Autodesk Fusion 360 part; units mm, degrees
sketch "Sketch1" plane through (0, 0, 0) normal (0, 1, 0) x (1, 0, 0)
  line L0 (-300, 30.15) -> (274, 30.15)
  line L1 (274, 30.15) -> (274, -30.15)
  line L2 (274, -30.15) -> (-300, -30.15)
  line L3 (-300, -30.15) -> (-300, 30.15)
  dimension "d1" = 574
  dimension "d2" = 60.3
  dimension "d3" = 300
  dimension "d4" = 30.15
extrude "Extrude1" add sketch "Sketch1" along normal blind 12
sketch "Sketch2" plane through (0, 12, 0) normal (0, 1, 0) x (-1, 0, 0)
  circle A0 centre (256.6, 26.25) radius 2
  line L0 (300, 30.15) -> (-274, 30.15)
  line L1 (300, -30.15) -> (300, 30.15)
  line L2 (256.6, 26.25) -> (294.4, 26.25) construction
  line L3 (294.4, 26.25) -> (294.4, -26.25) construction
  line L4 (294.4, -26.25) -> (256.6, -26.25) construction
  line L5 (256.6, -26.25) -> (256.6, 26.25) construction
  circle A1 centre (294.4, -26.25) radius 2
  circle A2 centre (256.6, -26.25) radius 2
  circle A3 centre (294.4, 26.25) radius 2
  dimension "d9" = 4
  dimension "d13" = 52.5
  dimension "d14" = 37.8
  dimension "d15" = 26.25
  dimension "d16" = 5.6
  dimension "d17" = 4
  dimension "d18" = 4
  dimension "d19" = 4
extrude "Extrude2" cut sketch "Sketch2" against normal through all
sketch "Sketch3" plane through (0, 12, 0) normal (0, 1, 0) x (-1, 0, 0)
  circle A0 centre (256.6, 26.25) radius 2
  line L0 (300, 30.15) -> (-274, 30.15)
  line L1 (-274, 30.15) -> (-274, -30.15)
  line L2 (-274, -30.15) -> (300, -30.15)
  line L3 (300, -30.15) -> (300, 30.15)
  circle A1 centre (256.6, -26.25) radius 2
  circle A2 centre (294.4, -26.25) radius 2
  circle A3 centre (294.4, 26.25) radius 2
sketch "Sketch4" plane through (0, 12, 0) normal (0, 1, 0) x (-1, 0, 0)
  line L0 (300, 30.15) -> (-274, 30.15)
  line L1 (-274, 30.15) -> (-274, -30.15)
  line L2 (-274, -30.15) -> (300, -30.15)
  line L3 (300, -30.15) -> (300, 30.15)
  circle A0 centre (256.6, -26.25) radius 2
  circle A1 centre (294.4, -26.25) radius 2
  circle A2 centre (256.6, 26.25) radius 2
  circle A3 centre (294.4, 26.25) radius 2
  circle A4 centre (-270, -26.25) radius 2
  circle A5 centre (-270, 26.25) radius 2
  dimension "d21" = 4
  dimension "d22" = 4
  dimension "d23" = 52.5
  dimension "d26" = 4
  dimension "d27" = 4
  dimension "d30" = 26.25
extrude "Extrude4" cut sketch "Sketch4" against normal through all contours A4 | A5
sketch "Sketch5" plane through (0, 12, 0) normal (0, 1, 0) x (-1, 0, 0)
  circle A0 centre (-270, -26.25) radius 2
  circle A1 centre (-270, 26.25) radius 2
  line L0 (-274, -30.15) -> (300, -30.15)
  line L1 (300, -30.15) -> (300, 30.15)
  line L2 (300, 30.15) -> (-274, 30.15)
  line L3 (-274, 30.15) -> (-274, -30.15)
  circle A2 centre (256.6, -26.25) radius 2
  circle A3 centre (294.4, -26.25) radius 2
  circle A4 centre (256.6, 26.25) radius 2
  circle A5 centre (294.4, 26.25) radius 2
  line L4 (240, 0) -> (-260, 0) construction
  circle A6 centre (230, 0) radius 1.5
  circle A7 centre (205, 0) radius 1.5
  circle A8 centre (180, 0) radius 1.5
  circle A9 centre (155, 0) radius 1.5
  circle A10 centre (130, 0) radius 1.5
  circle A11 centre (105, 0) radius 1.5
  circle A12 centre (80, 0) radius 1.5
  circle A13 centre (55, 0) radius 1.5
  circle A14 centre (30, 0) radius 1.5
  circle A15 centre (5, 0) radius 1.5
  circle A16 centre (-20, 0) radius 1.5
  circle A17 centre (-45, 0) radius 1.5
  circle A18 centre (-70, 0) radius 1.5
  circle A19 centre (-95, 0) radius 1.5
  circle A20 centre (-120, 0) radius 1.5
  circle A21 centre (-145, 0) radius 1.5
  circle A22 centre (-170, 0) radius 1.5
  circle A23 centre (-195, 0) radius 1.5
  circle A24 centre (-220, 0) radius 1.5
  circle A25 centre (-245, 0) radius 1.5
  dimension "d34" = 60
  dimension "d35" = 10
  dimension "d36" = 3
  dimension "d39" = -25
  dimension "d40" = 0
  dimension "d41" = 500
  dimension "d42" = 25
  dimension "d43" = 15
extrude "Extrude5" cut sketch "Sketch5" against normal through all contours A6 | A7 | A8 | A9 | A10 | A11 | A12 | A13 | A14 | A15 | A16 | A17 | A18 | A19 | A20 | A21 | A22 | A23 | A24 | A25
sketch "Sketch6" plane through (0, 0, 0) normal (0, -1, 0) x (1, 0, 0)
  circle A0 centre (195, 0) radius 1.5
  circle A1 centre (95, 0) radius 1.5
  circle A2 centre (-5, 0) radius 1.5
  circle A3 centre (-105, 0) radius 1.5
  circle A4 centre (-205, 0) radius 1.5
  circle A5 centre (-180, 0) radius 1.5
  circle A6 centre (-80, 0) radius 1.5
  circle A7 centre (20, 0) radius 1.5
  circle A8 centre (120, 0) radius 1.5
  circle A9 centre (220, 0) radius 1.5
  circle A10 centre (170, 0) radius 1.5
  circle A11 centre (70, 0) radius 1.5
  circle A12 centre (-30, 0) radius 1.5
  circle A13 centre (-130, 0) radius 1.5
  circle A14 centre (-230, 0) radius 1.5
  circle A15 centre (-155, 0) radius 1.5
  circle A16 centre (-55, 0) radius 1.5
  circle A17 centre (45, 0) radius 1.5
  circle A18 centre (145, 0) radius 1.5
  circle A19 centre (245, 0) radius 1.5
  circle A20 centre (270, -26.25) radius 2
  circle A21 centre (270, 26.25) radius 2
  circle A22 centre (-256.6, -26.25) radius 2
  circle A23 centre (-294.4, -26.25) radius 2
  circle A24 centre (-256.6, 26.25) radius 2
  circle A25 centre (-294.4, 26.25) radius 2
  line L0 (274, -30.15) -> (274, 30.15)
  line L1 (274, 30.15) -> (-300, 30.15)
  line L2 (-300, 30.15) -> (-300, -30.15)
  line L3 (-300, -30.15) -> (274, -30.15)
  line L4 (-292, 10) -> (-263, 10)
  line L5 (-260, 7) -> (-260, -7)
  line L6 (-263, -10) -> (-292, -10)
  line L7 (-295, -7) -> (-295, 7)
  arc A26 (-292, 10) -> (-295, 7) centre (-292, 7) ccw
  arc A27 (-260, 7) -> (-263, 10) centre (-263, 7) ccw
  arc A28 (-263, -10) -> (-260, -7) centre (-263, -7) ccw
  arc A29 (-295, -7) -> (-292, -10) centre (-292, -7) ccw
  dimension "d45" = 20.15
  dimension "d46" = 20
  dimension "d47" = 35
  dimension "d48" = 5
  dimension "d49" = 3
  dimension "d50" = 3
extrude "Extrude6" cut sketch "Sketch6" against normal through all contours L4 L5 L6 L7 A26 A27 A28 A29
sketch "Sketch8" plane through (0, 0, 0) normal (0, -1, 0) x (1, 0, 0)
  line L0 (-260, 7) -> (-260, -7)
  arc A0 (-263, -10) -> (-260, -7) centre (-263, -7) ccw
  line L1 (-263, -10) -> (-292, -10)
  arc A1 (-295, -7) -> (-292, -10) centre (-292, -7) ccw
  line L2 (-295, -7) -> (-295, 7)
  arc A2 (-292, 10) -> (-295, 7) centre (-292, 7) ccw
  line L3 (-292, 10) -> (-263, 10)
  arc A3 (-260, 7) -> (-263, 10) centre (-263, 7) ccw
  circle A4 centre (195, 0) radius 1.5
  circle A5 centre (95, 0) radius 1.5
  circle A6 centre (-5, 0) radius 1.5
  circle A7 centre (-105, 0) radius 1.5
  circle A8 centre (-205, 0) radius 1.5
  circle A9 centre (-180, 0) radius 1.5
  circle A10 centre (-80, 0) radius 1.5
  circle A11 centre (20, 0) radius 1.5
  circle A12 centre (120, 0) radius 1.5
  circle A13 centre (220, 0) radius 1.5
  circle A14 centre (170, 0) radius 1.5
  circle A15 centre (70, 0) radius 1.5
  circle A16 centre (-30, 0) radius 1.5
  circle A17 centre (-130, 0) radius 1.5
  circle A18 centre (-230, 0) radius 1.5
  circle A19 centre (-155, 0) radius 1.5
  circle A20 centre (-55, 0) radius 1.5
  circle A21 centre (45, 0) radius 1.5
  circle A22 centre (145, 0) radius 1.5
  circle A23 centre (245, 0) radius 1.5
  circle A24 centre (270, -26.25) radius 2
  circle A25 centre (270, 26.25) radius 2
  circle A26 centre (-256.6, -26.25) radius 2
  circle A27 centre (-294.4, -26.25) radius 2
  circle A28 centre (-256.6, 26.25) radius 2
  circle A29 centre (-294.4, 26.25) radius 2
  line L4 (274, -30.15) -> (274, 30.15)
  line L5 (274, 30.15) -> (-300, 30.15)
  line L6 (-300, 30.15) -> (-300, -30.15)
  line L7 (-300, -30.15) -> (274, -30.15)
  circle A30 centre (-230, 0) radius 1.5
  line L8 (-237.5, 3.05) -> (252.5, 3.05)
  line L9 (252.5, 3.05) -> (252.5, -3.05)
  line L10 (252.5, -3.05) -> (-237.5, -3.05)
  line L11 (-237.5, -3.05) -> (-237.5, 3.05)
  line L12 (242.25, 2.75) -> (247.75, 2.75) construction
  line L13 (247.75, 2.75) -> (247.75, -2.75) construction
  line L14 (247.75, -2.75) -> (242.25, -2.75) construction
  line L15 (242.25, -2.75) -> (242.25, 2.75) construction
  circle A31 centre (249.5, 0.05) radius 3 construction
  line L16 (-232.75, 2.75) -> (-227.25, 2.75) construction
  line L17 (-227.25, 2.75) -> (-227.25, -2.75) construction
  line L18 (-227.25, -2.75) -> (-232.75, -2.75) construction
  line L19 (-232.75, -2.75) -> (-232.75, 2.75) construction
  dimension "d54" = 490
  dimension "d55" = 6.1
  dimension "d56" = 3.05
  dimension "d57" = 7.5
  dimension "d64" = 5.5
  dimension "d65" = 5.5
  dimension "d66" = 2.75
  dimension "d67" = 2.75
  dimension "d68" = 6
  dimension "d69" = 90
  dimension "d70" = 90
  dimension "d71" = 90
  dimension "d72" = 90
  dimension "d73" = 5.5
  dimension "d74" = 2.75
  dimension "d75" = 5.5
  dimension "d76" = 2.75
extrude "Extrude7" cut sketch "Sketch8" against normal blind 3 contours L8 L9 L10 L11
extrude "Extrude8" cut 1 faces at (-235.5, 3, 0) along direction (0, 1, 0) blind 3
hole "Hole3" at (242.5, 0, 7) direction (0, 1, 0) diameter 3 depth 10 tip angle 180
hole "Hole4" at (-227.5, 0, 7) direction (0, 1, 0) diameter 3 depth 10 tip angle 180
hole "Hole5" at (242.5, 0, -7) direction (0, 1, 0) diameter 3 depth 10 tip angle 180
hole "Hole6" at (-227.5, 0, -7) direction (0, 1, 0) diameter 3 depth 10 tip angle 180
equation "d1 = 600 mm - 19 mm - 7 mm"
equation "d4 = ( 60.3 / 2 ) * 1 mm"
equation "d15 = ( 52.5 / 2 ) * 1 mm"
equation "d34 = 75 mm - 15 mm"
equation "d56 = ( 6.1 / 2 ) * 1 mm"
equation "d66 = ( 5.5 / 2 ) * 1 mm"
equation "d67 = ( 5.5 / 2 ) * 1 mm"
equation "d74 = ( 5.5 / 2 ) * 1 mm"
equation "d76 = ( 5.5 / 2 ) * 1 mm"
equation "dbToolDia = 3 mm"
equation "dbOffset = 0 mm"
equation "dbRadius = ( dbToolDia + dbOffset ) / 2"
equation "dbHoleOffset = dbRadius / sqrt(2)"
equation "d91 = dbRadius * 2"
equation "d93 = dbHoleOffset"
equation "d94 = dbHoleOffset"
equation "d96 = dbRadius * 2"
equation "d98 = dbHoleOffset"
equation "d99 = dbHoleOffset"
equation "d101 = dbRadius * 2"
equation "d103 = dbHoleOffset"
equation "d104 = dbHoleOffset"
equation "d106 = dbRadius * 2"
equation "d108 = dbHoleOffset"
equation "d109 = dbHoleOffset"
Design review of the part built by this model. Coordinates are the model's own, in mm. A direction names the side the tool comes from. Coordinates: 2 decimals unless noted, no trailing zeros. Order: outer loops, then holes, each group sorted by start corner. A loop starts at its lowest first (then second) coordinate and runs counter-clockwise, first axis right, second up. Notation, with made-up numbers: (89.25, -8) -> (136.25, -8) arc R30 ccw to (136.25, 20) -> close; hole circle Ø6 at (76.5, 40.25). An arc over 180 degrees is marked (long way). One line per item, written item: value. Start each with the question number.
Q1. Take a section at B-B, the plane x = 204.5. State the section outline as (y, z) points, then the cut area to 3 significant figures.
Q2. Mouldability with a two-part tool opening along X and no side actions: class faces 3 (the flat face through (-9, 6, 30.15)), 4 (the flat face through (-300, 6, 0)), 5 (the flat face through (-278, 6, 10)) as pulls with the +X half, pulls with the -X half, needs draft (parallel to the pull), parting line crosses it, or undercut.
Q3. Insertion check: pin 1 Ø1.5 at (x, z) = (2, 1.5) entering from -Y; pin 2 Ø2.5 at (x, z) = (145, 0) entering from +Y. Each pin has a flat end and moves straight along its axis. Give the tip position at first contact, or say it passes through.
Q4. Tool access review of faces 1 (the flat face through (-17, 0, -7)), 2 (the flat face through (-295, 6, 0)): name each direction out of +Z, -Z, +X, -X, +Y, -Y from which nothing blocks a thin tool from reaching the whole face with its end or side.
Q5. Take a section at A-A, the plane y = 3.5. Give the number of separate pieces and of enclosed holes in the cut face, then the cut area to 3 significant figures.
Q6. For probe 1 along Z at (x, y) = (242.5, 5); probe 2 along X at (y, z) = (7.5, 7); probe 3 along X at (y, z) = (2.75, 3), list the stretches that pass through material, from the lowest coordinate up.
Values follow:
1. outline: (0, -30.15) -> (12, -30.15) -> (12, 30.15) -> (0, 30.15) -> (0, 3.05) -> (6, 3.05) -> (6, -3.05) -> (0, -3.05) -> close
1. area: 687 mm2
2. face 3: needs draft
2. face 4: pulls with the -X half
2. face 5: undercut
3. pin 1: stops at y = 6
3. pin 2: passes through
4. face 1: +Z, -Z, +X, -X, -Y
4. face 2: +Y, -Y
5. separate pieces: 1
5. enclosed holes: 12
5. area: 30,800 mm2
6. probe 1: z = -30.15 to -8.5, -5.5 to -3.05, 3.05 to 5.5, 8.5 to 30.15
6. probe 2: x = -300 to -295, -260 to -229, -226 to 241, 244 to 274
6. probe 3: x = -300 to -295, -260 to -237.5, 252.5 to 274
